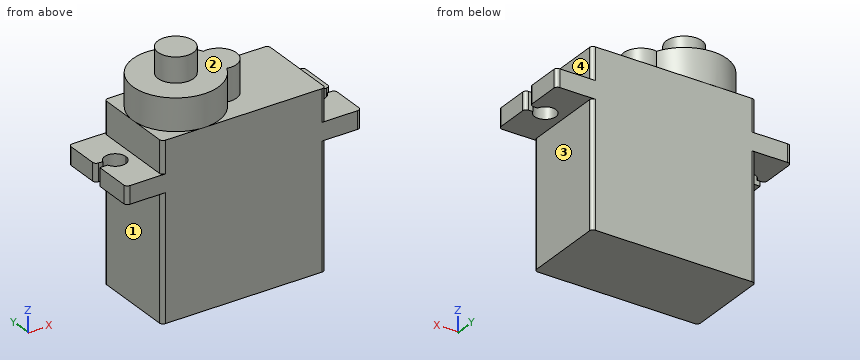
from build123d import *

# Parameters (mm, degrees)
ESQUISSE1_W             = 23
ESQUISSE1_H             = 12
BOSS_EXTRU_1_DEPTH      = 17.5
ESQUISSE2_W             = 33
ESQUISSE2_H             = 12
BOSS_EXTRU_2_DEPTH      = 2.5
ESQUISSE3_W             = 23
ESQUISSE3_H             = 12
BOSS_EXTRU_3_DEPTH      = 4.5
ESQUISSE4_R             = 6.022589187
BOSS_EXTRU_4_DEPTH      = 4.5
ESQUISSE5_R             = 2.5
BOSS_EXTRU_5_DEPTH      = 4.5
ESQUISSE6_R             = 2.5
BOSS_EXTRU_6_DEPTH      = 3.5
ENL_V_MAT_EXTRU_3_DEPTH = 21
CONG_2_R                = 0.5


with BuildPart() as part:
    # Esquisse1 → Boss.-Extru.1 (new body)
    with BuildSketch(Plane.XY):
        with Locations((-4.910575451, 4.41260745)):
            Rectangle(ESQUISSE1_W, ESQUISSE1_H)
    extrude(amount=BOSS_EXTRU_1_DEPTH)

    # Esquisse2 → Boss.-Extru.2 (add)
    with BuildSketch(Plane.XY.offset(17.5)):
        with Locations((-4.910575451, 4.41260745)):
            Rectangle(ESQUISSE2_W, ESQUISSE2_H)
    extrude(amount=BOSS_EXTRU_2_DEPTH)

    # Esquisse3 → Boss.-Extru.3 (add)
    with BuildSketch(Plane.XY.offset(20)):
        with Locations((-4.910575451, 4.41260745)):
            Rectangle(ESQUISSE3_W, ESQUISSE3_H)
    extrude(amount=BOSS_EXTRU_3_DEPTH)

    # Esquisse4 → Boss.-Extru.4 (add)
    with BuildSketch(Plane.XY.offset(24.5)):
        with Locations((-10.410575451, 4.41260745)):
            Circle(ESQUISSE4_R)
    extrude(amount=BOSS_EXTRU_4_DEPTH)

    # Esquisse5 → Boss.-Extru.5 (add)
    with BuildSketch(Plane.XY.offset(24.5)):
        with Locations((-4.387986264, 4.41260745)):
            Circle(ESQUISSE5_R)
    extrude(amount=BOSS_EXTRU_5_DEPTH)

    # Esquisse6 → Boss.-Extru.6 (add)
    with BuildSketch(Plane.XY.offset(29)):
        with Locations((-10.410575451, 4.41260745)):
            Circle(ESQUISSE6_R)
    extrude(amount=BOSS_EXTRU_6_DEPTH)

    # Esquisse7 → Enlèv. mat.-Extru.3 (cut, through all)
    with BuildSketch(Plane.XY.offset(20)):
        with BuildLine():
            ThreePointArc((-20.324789014, 4.91260745), (-20.410575451, 4.41260745), (-20.324789014, 3.91260745))
            Line((-20.324789014, 3.91260745), (-20.324789014, 4.91260745))
        make_face()
        with BuildLine():
            Line((-20.324789014, 4.91260745), (-20.324789014, 3.91260745))
            ThreePointArc((-20.324789014, 3.91260745), (-18.656922483, 2.93420961), (-17.410575451, 4.41260745))
            ThreePointArc((-17.410575451, 4.41260745), (-18.656922483, 5.891005289), (-20.324789014, 4.91260745))
        make_face()
        with BuildLine():
            Line((-21.410575451, 4.91260745), (-21.410575451, 3.91260745))
            Line((-21.410575451, 3.91260745), (-20.324789014, 3.91260745))
            ThreePointArc((-20.324789014, 3.91260745), (-20.410575451, 4.41260745), (-20.324789014, 4.91260745))
            Line((-20.324789014, 4.91260745), (-21.410575451, 4.91260745))
        make_face()
        with BuildLine():
            ThreePointArc((10.589424549, 4.41260745), (10.567822388, 4.666260418), (10.503638111, 4.91260745))
            Line((10.503638111, 4.91260745), (10.503638111, 3.91260745))
            ThreePointArc((10.503638111, 3.91260745), (10.567822388, 4.158954482), (10.589424549, 4.41260745))
        make_face()
        with BuildLine():
            Line((10.503638111, 3.91260745), (10.503638111, 4.91260745))
            ThreePointArc((10.503638111, 4.91260745), (7.589424549, 4.41260745), (10.503638111, 3.91260745))
        make_face()
        with BuildLine():
            Line((12.675210986, 3.91260745), (12.675210986, 4.91260745))
            Line((12.675210986, 4.91260745), (10.503638111, 4.91260745))
            ThreePointArc((10.503638111, 4.91260745), (10.567822388, 4.666260418), (10.589424549, 4.41260745))
            ThreePointArc((10.589424549, 4.41260745), (10.567822388, 4.158954482), (10.503638111, 3.91260745))
            Line((10.503638111, 3.91260745), (12.675210986, 3.91260745))
        make_face()
    extrude(amount=-ENL_V_MAT_EXTRU_3_DEPTH, mode=Mode.SUBTRACT)

    # Congé2
    cong_2_edges = [part.edges().sort_by_distance(p)[0] for p in [
        (-21.410575451, 10.41260745, 18.75),
        (-21.410575451, -1.58739255, 18.75),
        (11.589424549, -1.58739255, 18.75),
        (11.589424549, 10.41260745, 18.75),
        (-16.410575451, 10.41260745, 22.25),
        (-16.410575451, -1.58739255, 22.25),
        (6.589424549, -1.58739255, 22.25),
        (6.589424549, 10.41260745, 22.25),
        (-21.410575451, 4.91260745, 18.75),
        (-16.410575451, 10.41260745, 8.75),
        (6.589424549, 10.41260745, 8.75),
        (6.589424549, -1.58739255, 8.75),
        (-16.410575451, -1.58739255, 8.75),
        (11.589424549, 4.91260745, 18.75),
        (11.589424549, 3.91260745, 18.75),
    ]]
    fillet(cong_2_edges, radius=CONG_2_R)


solid = part.part
Read the model definition and answer for the solid it produces. Units are mm, in the model's axes. Face numbers are marked on the shaded views. A direction names the side the tool comes from. Round coordinates to 2 decimals unless told otherwise and drop trailing zeros. Write each loop counter-clockwise with the first axis right and the second up, starting at its lowest first coordinate (ties: lowest second). Pieces come first, ordered by that corner, then holes.
1. The part is cut by section D-D, the plane y = 1.5. Determine the outline of the cut face in (x, z).
2. The part is cut by section B-B, the plane z = 2. Determine the outline of the cut face in (x, y), then the cut area to 3 significant figures.
3. Which of the six approach directions +Z, -Z, +X, -X, +Y, -Y give full straight-line access (tool end or side, diameter ignored) to the marked faces 1, 2, 3 and 4?
4. Straight lines are drawn through the part: L1, parallel to Z at x = 9, y = 10; L2, parallel to Y at x = 2.5, z = 17.5; L3, parallel to Z at x = -15, y = 6. For each, find the intervals that lie inside material, in ascending order.
5. The part is cut by section A-A, the plane x = 8. Determine the outline of the cut face in (y, z).
6. Given pin 1 Ø1 at (x, y) = (-5, -0.5) entering from +Z; pin 2 Ø2 at (x, z) = (-1.5, 17.5) entering from -Y; pin 3 Ø1.6 at (x, y) = (-14, 7.5) entering from +Z, each flat-ended and moving along its own axis, determine where each tip first touches the part or whether it passes through.
7. The part is cut by section C-C, the plane x = -3. Determine the outline of the cut face in (y, z).
Values:
1. outline: (-21.41, 17.5) - (-16.41, 17.5) - (-16.41, 0) - (6.59, 0) - (6.59, 17.5) - (11.59, 17.5) - (11.59, 20) - (6.59, 20) - (6.59, 24.5) - (-5.14, 24.5) - (-5.14, 29) - (-15.68, 29) - (-15.68, 24.5) - (-16.41, 24.5) - (-16.41, 20) - (-21.41, 20) - close
2. outline: (-16.41, -1.09) arc R0.5 ccw to (-15.91, -1.59) - (6.09, -1.59) arc R0.5 ccw to (6.59, -1.09) - (6.59, 9.91) arc R0.5 ccw to (6.09, 10.41) - (-15.91, 10.41) arc R0.5 ccw to (-16.41, 9.91) - close
2. area: 276 mm2
3. face 1: -Z, -X, +Y, -Y
3. face 2: +Z
3. face 3: -Z, +X, +Y, -Y
3. face 4: +Z, +X, +Y, -Y
4. L1: z = 17.5 to 20
4. L2: y = -1.59 to 10.41
4. L3: z = 0 to 29
5. outline: (-1.59, 17.5) - (3.38, 17.5) - (3.38, 20) - (-1.59, 20) - close; (5.44, 17.5) - (10.41, 17.5) - (10.41, 20) - (5.44, 20) - close
6. pin 1: stops at z = 24.5
6. pin 2: stops at y = -1.59
6. pin 3: stops at z = 29
7. outline: (-1.59, 0) - (10.41, 0) - (10.41, 24.5) - (6.49, 24.5) - (6.49, 29) - (2.33, 29) - (2.33, 24.5) - (-1.59, 24.5) - close
